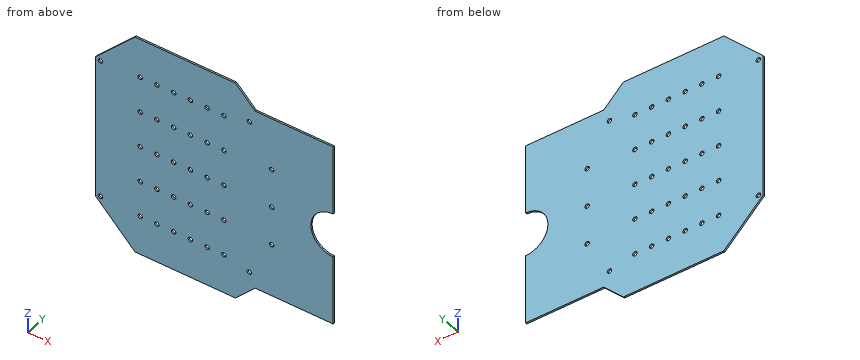
from build123d import *

# Parameters (mm, degrees)
Y_KSEKLIK_EKSTR_ZYON1_DEPTH = 1.5
IZIM2_R                     = 2
KES_EKSTR_ZYON1_DEPTH       = 10
IZIM3_R                     = 2
KES_EKSTR_ZYON2_DEPTH       = 10
IZIM4_R                     = 20
KES_EKSTR_ZYON3_DEPTH       = 10


with BuildPart() as part:
    # Çizim1 → Yükseklik-Ekstrüzyon1 (new body)
    with BuildSketch(Plane(origin=(0, 0, 0), x_dir=(1, 0, 0), z_dir=(0, 1, 0))):
        Polygon((-27.784830075, -18.817907641), (-27.784830075, 111.182092359), (7.570508985, 146.537431418), (97.570508985, 146.537431418), (115.248178514, 128.859761888), (185.248178514, 128.859761888), (185.248178514, -36.495577171), (115.248178514, -36.495577171), (97.570508985, -54.173246701), (7.570508985, -54.173246701), align=None)
    extrude(amount=Y_KSEKLIK_EKSTR_ZYON1_DEPTH)

    # Çizim2 → Kes-Ekstrüzyon1 (cut)
    with BuildSketch(Plane(origin=(0, 1.5, 0), x_dir=(1, 0, 0), z_dir=(0, 1, 0))):
        with Locations(Location((-23.433357477, 109.379653392, 0), (0, 0, 270))):
            Circle(IZIM2_R)
        with Locations(Location((-23.433357477, -17.015468675, 0), (0, 0, 270))):
            Circle(IZIM2_R)
        with Locations(Location((110.070471674, -23.995487096, 0), (0, 0, 270))):
            Circle(IZIM2_R)
        with Locations(Location((110.070471674, 116.359671813, 0), (0, 0, 270))):
            Circle(IZIM2_R)
        with Locations(Location((130.070471674, 46.182092359, 0), (0, 0, 270))):
            Circle(IZIM2_R)
        with Locations(Location((130.070471674, 81.270882086, 0), (0, 0, 270))):
            Circle(IZIM2_R)
        with Locations(Location((130.070471674, 11.093302631, 0), (0, 0, 270))):
            Circle(IZIM2_R)
    extrude(amount=-KES_EKSTR_ZYON1_DEPTH, mode=Mode.SUBTRACT)

    # Çizim3 → Kes-Ekstrüzyon2 (cut)
    with BuildSketch(Plane(origin=(0, 1.5, 0), x_dir=(1, 0, 0), z_dir=(0, 1, 0))):
        with Locations(Location((12.215169925, 46.182092359, 0), (0, 0, 270))):
            Circle(IZIM3_R)
        with Locations(Location((12.215169925, 78.682092359, 0), (0, 0, 270))):
            Circle(IZIM3_R)
        with Locations(Location((12.215169925, 13.682092359, 0), (0, 0, 270))):
            Circle(IZIM3_R)
        with Locations(Location((27.215169925, 78.682092359, 0), (0, 0, 270))):
            Circle(IZIM3_R)
        with Locations(Location((42.215169925, 78.682092359, 0), (0, 0, 270))):
            Circle(IZIM3_R)
        with Locations(Location((57.215169925, 78.682092359, 0), (0, 0, 270))):
            Circle(IZIM3_R)
        with Locations(Location((72.215169925, 78.682092359, 0), (0, 0, 270))):
            Circle(IZIM3_R)
        with Locations(Location((87.215169925, 78.682092359, 0), (0, 0, 270))):
            Circle(IZIM3_R)
        with Locations(Location((27.215169925, 46.182092359, 0), (0, 0, 270))):
            Circle(IZIM3_R)
        with Locations(Location((42.215169925, 46.182092359, 0), (0, 0, 270))):
            Circle(IZIM3_R)
        with Locations(Location((57.215169925, 46.182092359, 0), (0, 0, 270))):
            Circle(IZIM3_R)
        with Locations(Location((72.215169925, 46.182092359, 0), (0, 0, 270))):
            Circle(IZIM3_R)
        with Locations(Location((87.215169925, 46.182092359, 0), (0, 0, 270))):
            Circle(IZIM3_R)
        with Locations(Location((27.215169925, 13.682092359, 0), (0, 0, 270))):
            Circle(IZIM3_R)
        with Locations(Location((42.215169925, 13.682092359, 0), (0, 0, 270))):
            Circle(IZIM3_R)
        with Locations(Location((57.215169925, 13.682092359, 0), (0, 0, 270))):
            Circle(IZIM3_R)
        with Locations(Location((72.215169925, 13.682092359, 0), (0, 0, 270))):
            Circle(IZIM3_R)
        with Locations(Location((87.215169925, 13.682092359, 0), (0, 0, 270))):
            Circle(IZIM3_R)
        with Locations(Location((12.215169925, -18.817907641, 0), (0, 0, 270))):
            Circle(IZIM3_R)
        with Locations(Location((12.215169925, 111.182092359, 0), (0, 0, 270))):
            Circle(IZIM3_R)
        with Locations(Location((27.215169925, 111.182092359, 0), (0, 0, 270))):
            Circle(IZIM3_R)
        with Locations(Location((42.215169925, 111.182092359, 0), (0, 0, 270))):
            Circle(IZIM3_R)
        with Locations(Location((57.215169925, 111.182092359, 0), (0, 0, 270))):
            Circle(IZIM3_R)
        with Locations(Location((72.215169925, 111.182092359, 0), (0, 0, 270))):
            Circle(IZIM3_R)
        with Locations(Location((87.215169925, 111.182092359, 0), (0, 0, 270))):
            Circle(IZIM3_R)
        with Locations(Location((27.215169925, -18.817907641, 0), (0, 0, 270))):
            Circle(IZIM3_R)
        with Locations(Location((42.215169925, -18.817907641, 0), (0, 0, 270))):
            Circle(IZIM3_R)
        with Locations(Location((57.215169925, -18.817907641, 0), (0, 0, 270))):
            Circle(IZIM3_R)
        with Locations(Location((72.215169925, -18.817907641, 0), (0, 0, 270))):
            Circle(IZIM3_R)
        with Locations(Location((87.215169925, -18.817907641, 0), (0, 0, 270))):
            Circle(IZIM3_R)
    extrude(amount=-KES_EKSTR_ZYON2_DEPTH, mode=Mode.SUBTRACT)

    # Çizim4 → Kes-Ekstrüzyon3 (cut)
    with BuildSketch(Plane(origin=(0, 1.5, 0), x_dir=(1, 0, 0), z_dir=(0, 1, 0))):
        with Locations((185.248178514, 46.182092359)):
            Circle(IZIM4_R)
    extrude(amount=-KES_EKSTR_ZYON3_DEPTH, mode=Mode.SUBTRACT)


solid = part.part
Design review of the part built by this model. Coordinates are the model's own, in mm. Round coordinates to 2 decimals unless told otherwise and drop trailing zeros. Loops run counter-clockwise (first coordinate to the right, second up) from the corner with the lowest first, then second, coordinate; pieces in that order, holes last. Notation, with made-up numbers: (-29, 79.25) -> (-14, 79.25) arc R23 cw to (-14, 92.25) -> close; hole circle Ø5 at (20.5, 81). An arc over 180 degrees is marked (long way). Use one line per item in the form item = value. Start each with the question number.
Q1. We need section C-C on z = 33. Give the boundary of the cut face in (x, y).
Q2. We need section A-A on x = 134.5. Give the boundary of the cut face in (y, z), then the cut area to 3 significant figures.
Q3. Wall thickness on line 1 along Z through (x, y) = (168, 0.15); line 2 along Z through (x, y) = (134.5, 1.35); line 3 along Z through (x, y) = (44, 1.15): over which ranges is each line inside the solid? List them lowest first. Write a range as [from, to].
Q4. We need section B-B on y = 1.1. State how many separate pieces and enclosed holes the cut face has, then the cut area to 3 significant figures.
Q5. For pin 1 Ø3.5 at (x, z) = (130.07, -46.18) entering from +Y, flat-tipped, find the tip position at first contact; note if it passes through.
Calculated:
q1.outline = (-13.6, 0) -> (185.25, 0) -> (185.25, 1.5) -> (-13.6, 1.5) -> close
q2.outline = (0, -128.86) -> (1.5, -128.86) -> (1.5, 36.5) -> (0, 36.5) -> close
q2.area = 248 mm²
q3.line_1 = [-128.86, -56.31], [-36.06, 36.5]
q3.line_2 = [-128.86, 36.5]
q3.line_3 = [-146.54, -112.08], [-110.28, -79.58], [-77.78, -47.08], [-45.28, -14.58], [-12.78, 17.92], [19.72, 54.17]
q4.separate_pieces = 1
q4.enclosed_holes = 37
q4.area = 37,600 mm²
q5.pin_1 = through
